Geometry: final body of the model. Coordinates: model frame, mm. A direction names the side the tool comes from. Coordinates: 2 decimals unless noted, no trailing zeros. Order: outer loops, then holes, each group sorted by start corner. A loop starts at its lowest first (then second) coordinate and runs counter-clockwise, first axis right, second up. Notation, with made-up numbers: M 88.5,79.25 L 104.5,79.25 A18 cw 104.5,86.25 Z; hole C 58,-8 d4. An arc over 180 degrees is marked long. Write item = value, one per line.
Autodesk Inventor part; units mm, degrees
ref_plane "YZ Plane" through (0, 0, 0) normal (1, 0, 0) x (0, 1, 0)
ref_plane "XZ Plane" through (0, 0, 0) normal (0, 1, 0) x (-1, 0, 0)
ref_plane "XY Plane" through (0, 0, 0) normal (0, 0, 1) x (1, 0, 0)
sketch "Sketch1" plane through (0, 0, 0) normal (0, 0, 1) x (1, 0, 0)
  circle A0 centre (0, 0) radius 4.6
  dimension "d0" = 9.2
extrude "Extrusion1" add sketch "Sketch1" along normal blind 1
sketch "Sketch2" plane through (0, 0, 1) normal (0, 0, 1) x (1, 0, 0)
  circle A0 centre (0, 0) radius 4.05
  dimension "d3" = 8.1
extrude "Extrusion2" add sketch "Sketch2" along normal blind 3.2
sketch "Sketch3" plane through (0, 0, 0) normal (0, 0, -1) x (-1, 0, 0)
  line L0 (0, 0) -> (0, -4.6024)
  line L1 (0, -4.6024) -> (-0.5737, -4.5641)
  circle A0 centre (0, 0) radius 4.6
  line L2 (-0.5737, -4.5641) -> (0.5763, -4.5638)
  line L3 (0.5763, -4.5638) -> (0.5766, -5.5638)
  line L4 (0.5766, -5.5638) -> (-0.5734, -5.5641)
  line L5 (-0.5734, -5.5641) -> (-0.5737, -4.5641)
  dimension "d6" = 0.575
  dimension "d7" = 1.15
  dimension "d8" = 1
extrude "Extrusion3" add sketch "Sketch3" against normal blind 1 contours A0 L3 L4 L5 L1
fillet "Fillet1" radius 0.25 4 edges at (0.5737, -4.5641, 0.5) (0.5734, -5.5641, 0.5) (-0.5763, -4.5638, 0.5) (-0.5766, -5.5638, 0.5)
properties part number "sensor"
1) Section B-B, the plane x = 1. Return loops of the section in (y, z), and give its area (3 significant figures).
Numbers:
outline = M -4.49,0 L 4.49,0 L 4.49,1 L 3.92,1 L 3.92,4.2 L -3.92,4.2 L -3.92,1 L -4.49,1 Z
area = 34.1 mm²
2) Section A-A, the plane y = -3.75. Return loops of the section in (x, z), and give its area (3 significant figures).
Numbers:
outline = M -2.66,0 L 2.66,0 L 2.66,1 L 1.53,1 L 1.53,4.2 L -1.53,4.2 L -1.53,1 L -2.66,1 Z
area = 15.1 mm²
3) Section C-C, the plane z = 3.55. Return loops of the section in (x, y), and give its area (3 significant figures).
Numbers:
outline = C 0,0 d8.1
area = 51.5 mm²
4) Line query: L1, parallel to Z at x = -4, y = -2; L2, parallel to X at y = -5, z = 0.3; L3, parallel to Y at x = -1, z = 0.8. Output: solid intervals per line, ascending.
Numbers:
L1 = 0 to 1
L2 = -0.58 to 0.57
L3 = -4.49 to 4.49
5) Pin query (flat end, axial travel): pin 1 (1 mm diameter, centred on y = 3, z = 3, fed in from -X); pin 2 (2 mm diameter, centred on x = 3, z = 1, fed in from +Y); pin 3 (1.1 mm diameter, centred on x = -0.5, y = -5, fed in from +Z). Return the tip coordinate at first contact, or that it passes through.
Numbers:
pin_1 = -3.19
pin_2 = 4.14
pin_3 = 1
6) Set-up query: faces 1 (the face through (0, 0, 4.2)), 2 (the face through (-0.878, 3.954, 2.578)). Return all of +Z, -Z, +X, -X, +Y, -Y with unobstructed straight access to the full face (end or side cutting, diameter ignored); none if empty.
Numbers:
face_1 = +Z, +X, -X, +Y, -Y
face_2 = +Z
